Geometry check sheet. Reference: the model listing, model coordinates, mm. A direction names the side the tool comes from. Give positions to 0.01 mm unless a question says otherwise; leave off trailing zeros. Order: outer loops, then holes, each group sorted by start corner. A loop starts at its lowest first (then second) coordinate and runs counter-clockwise, first axis right, second up. Notation, with made-up numbers: M 63,34 L 76,34 A24 ccw 76,71 Z; hole C 65,87 d8. An arc over 180 degrees is marked long. Answer as CSV lines item,"result". Start each with the question number.
Q1. Section check A-A, the plane x = 0. Record the boundary of the cut face in (y, z).
Q2. Mould release check, pull along Y, two halves, no side actions. Record for faces 1 (the flat face through (144, -3, 12.5)), 2 (the cylindrical face through (-6, 0, 12)), 3 (the cylindrical face through (132.835, 7.154, 2.253)): +Y half, -Y half, draft (parallel to the pull), parting line (faces both ways), or undercut.
Q3. Thickness scan on line 1 (Y direction, x = 150, z = -5); line 2 (Y direction, x = 0, z = 16.25); line 3 (Z direction, x = 141, y = -1.5). Record the ranges inside material, lowest first.
Q4. Section check C-C, the plane z = 1.5. Count the separate pieces of the cut face and the enclosed holes in it, then the cut area to 3 significant figures.
Q5. Set-up check for faces 4 (the cylindrical face through (17.6, 6.93, 9.13)), 5 (the flat face through (-3, -5.4, 0)), 6 (the flat face through (144, -3, -12.5)): record each of +Z, -Z, +X, -X, +Y, -Y from which the full face is reachable in a straight line by a thin tool's end or side.
Q6. Section check D-D, the plane y = 9.5. Record the boundary of the cut face in (x, z).
Q7. Go/stop test with flat-tipped pins: pin 1 (5 mm diameter, centred on x = 57, z = 5.5, fed in from -Y); pin 2 (2 mm diameter, centred on x = 10, z = 19, fed in from +Y); pin 3 (5 mm diameter, centred on x = 74.5, y = -0.5, fed in from -Z). Record where each tip stops, or that it passes through.
Q8. Section check B-B, the plane y = 0. Record the boundary of the cut face in (x, z), then the cut area to 3 significant figures.
```python
from build123d import *

# Parameters (mm, degrees)
F0_R          = 12.5
F1_DEPTH      = 25
F0_R_2        = 12.1407528782
F2_DEPTH      = 12.5
F4_R          = 7.5
F6_R          = 6
F7_DEPTH      = 12.5010001
F7_DEPTH_BACK = 25.0010001


with BuildPart() as f1:
    # F0 (on Top) → F1 (new body)
    with BuildSketch(Plane.XY):
        Circle(F0_R)
    extrude(amount=F1_DEPTH)



with BuildPart() as f2:
    # F0 (on Top) → F2 (new body, symmetric)
    with BuildSketch(Plane.XY):
        with Locations((150, 0)):
            Circle(F0_R_2)
    extrude(amount=F2_DEPTH, both=True)


with BuildPart() as f1_1:
    add(f1.part)

    add(f2.part)  # F5 merges F2
    # F5: sweep along a path in F3
    with BuildLine(Plane.XZ) as f5_path:
        Line((0, 12), (25, 12))
        ThreePointArc((25, 12), (32.1487132371, 11.5726103092), (39.1955835962, 10.2965299685))
        ThreePointArc((39.1955835962, 10.2965299685), (81.789999989, 2.5833332421), (125, 0))
        Line((125, 0), (150, 0))
    # F4 (on Right) → F5 (sweep)
    with BuildSketch(Plane.YZ):
        with Locations((0, 12)):
            Circle(F4_R)
    sweep(path=f5_path.line)

    # F6 (on Top) → F7 (cut, two sides)
    with BuildSketch(Plane.XY) as f7_sk:
        Circle(F6_R)
        with Locations((150, 0)):
            Circle(F6_R)
    extrude(amount=-F7_DEPTH, mode=Mode.SUBTRACT)
    extrude(f7_sk.sketch, amount=F7_DEPTH_BACK, mode=Mode.SUBTRACT)


solid = f1_1.part
```
Answer block:
1,outline,"M -12.5,0 L -6,0 L -6,25 L -12.5,25 Z; M 6,0 L 12.5,0 L 12.5,25 L 6,25 Z"
2,face 1,"draft"
2,face 2,"undercut"
2,face 3,"parting line"
3,line 1,"y = -12.14 to -6, 6 to 12.14"
3,line 2,"y = -12.5 to -6, 6 to 12.5"
3,line 3,"z = -12.5 to 12.5"
4,separate pieces,"2"
4,enclosed holes,"2"
4,area,"2,020 mm2"
5,face 4,"none"
5,face 5,"-Z, -X, +Y, -Y"
5,face 6,"-Z, +X, -X, +Y, -Y"
6,outline,"M -8.12,0 L 8.12,0 L 8.12,25 L -8.12,25 Z; M 142.44,-12.5 L 157.56,-12.5 L 157.56,12.5 L 142.44,12.5 Z"
7,pin 1,"stops at y = -7.5"
7,pin 2,"stops at y = 8.67"
7,pin 3,"stops at z = -4.37"
8,outline,"M -12.5,0 L -6,0 L -6,25 L -12.5,25 Z; M 6,0 L 12.5,0 L 12.5,4.5 L 25,4.5 A52.5 cw 37.42,3.01 A370.17 ccw 125,-7.5 L 137.86,-7.5 L 137.86,-12.5 L 144,-12.5 L 144,12.5 L 137.86,12.5 L 137.86,7.5 L 125,7.5 A355.17 cw 40.97,17.58 A67.5 ccw 25,19.5 L 12.5,19.5 L 12.5,25 L 6,25 Z; M 156,-12.5 L 162.14,-12.5 L 162.14,12.5 L 156,12.5 Z"
8,area,"2,530 mm2"
